The model under review builds one solid part; all positions refer to its coordinate system, in mm. Coordinates: 2 decimals unless noted, no trailing zeros. Write each loop counter-clockwise with the first axis right and the second up, starting at its lowest first coordinate (ties: lowest second). Pieces come first, ordered by that corner, then holes. Notation, with made-up numbers: (4, 22.25) - (23, 22.25) arc R19 ccw to (23, 31.25) - close; hole circle Ø5 at (58, -18.75). An arc over 180 degrees is marked (long way). Return JSON: item names as keys, results as strings. Group by question number.
(1) We need section A-A on z = 3.35. State the section outline as (x, y) points.
(2) We need section C-C on x = 47. State the section outline as (y, z) points.
(3) To check wall thickness, follow L1, parallel to Y at x = 65, z = 4.55; L2, parallel to Y at x = 109.5, z = 2.85; L3, parallel to X at y = -108, z = 3.4. State the ranges of each line that lie inside material, in increasing order. Write a range as from..to.
(4) We need section B-B on y = 101.5. State the section outline as (x, z) points.
(5) Draft analysis for pull direction Y (two halves, no side actions). For faces 1 (the face through (116, 13, 5)), 2 (the face through (50.7, 122.99, 2.54)), 3 (the face through (98.92, 14.67, 2.46)), state which applies: released by +Y, released by -Y, zero draft, split by the parting line, or undercut.
(6) For pin 1 Ø2 at (x, z) = (57, 4) entering from -Y; pin 2 Ø1 at (y, z) = (113, 2) entering from -X; pin 3 Ø1.5 at (x, z) = (78.5, 2) entering from +Y, all flat-tipped, find the tip position at first contact; note any pin that passes through.
```python
from build123d import *

# Parameters (mm, degrees)
BOSS_EXTRU_2_DEPTH      = 5
ENL_V_MAT_EXTRU_1_DEPTH = 10
ESQUISSE3_W             = 70.825033907
ESQUISSE3_H             = 52.172348309
ENL_V_MAT_EXTRU_2_DEPTH = 10
ESQUISSE4_R             = 2
ESQUISSE4_R_2           = 1.87013138
ENL_V_MAT_EXTRU_3_DEPTH = 10
ENL_V_MAT_EXTRU_4_DEPTH = 10


with BuildPart() as part:
    # Esquisse1 → Boss.-Extru.2 (new body)
    with BuildSketch(Plane.XY):
        with BuildLine():
            Line((-2, 166.988023523), (-2, 99.979998))
            ThreePointArc((-2, 99.979998), (100, 0), (-2, -99.979998))
            Line((-2, -99.979998), (-2, -166.988023523))
            ThreePointArc((-2, -166.988023523), (167, 0), (-2, 166.988023523))
        make_face()
    extrude(amount=BOSS_EXTRU_2_DEPTH)

    # Esquisse2 → Enlèv. mat.-Extru.1 (cut)
    with BuildSketch(Plane.XY.offset(5)):
        Polygon((29.390638032, 43.425593165), (38.112910781, 92.452182407), (63.648561005, 154.395144619), (68.028776979, 172.275239399), (-24.955464007, 192.914301625), (-14.988060504, 82.801476905), align=None)
        Polygon((56.192163409, 19.645406226), (29.390638032, 43.425593165), (-11.148286352, -184.437631398), (102.415881909, -156.025065414), (102.415881909, -133.007210905), (53.907034164, -84.226074749), align=None)
    extrude(amount=-ENL_V_MAT_EXTRU_1_DEPTH, mode=Mode.SUBTRACT)

    # Esquisse3 → Enlèv. mat.-Extru.2 (cut)
    with BuildSketch(Plane.XY.offset(5)):
        with Locations((-10.008332903, -121.270932698)):
            Rectangle(ESQUISSE3_W, ESQUISSE3_H)
    extrude(amount=-ENL_V_MAT_EXTRU_2_DEPTH, mode=Mode.SUBTRACT)

    # Esquisse4 → Enlèv. mat.-Extru.3 (cut)
    with BuildSketch(Plane.XY.offset(5)):
        with Locations((109.034633389, 14.54127648)):
            Circle(ESQUISSE4_R)
        with Locations((101.697400647, -41.92420186)):
            Circle(ESQUISSE4_R)
        with Locations((87.156124167, 67.11043153)):
            Circle(ESQUISSE4_R_2)
        with Locations((122.810902236, 94.564698974)):
            Circle(ESQUISSE4_R)
        with Locations((143.30088273, -59.075011711)):
            Circle(ESQUISSE4_R)
        with Locations((153.639710685, 20.489980494)):
            Circle(ESQUISSE4_R)
    extrude(amount=-ENL_V_MAT_EXTRU_3_DEPTH, mode=Mode.SUBTRACT)

    # Esquisse5 → Enlèv. mat.-Extru.4 (cut)
    with BuildSketch(Plane.XY.offset(5)):
        Polygon((61.009483209, -79.232840152), (101.798321541, -132.386184065), (46.643469874, -98.897205978), (43.215654561, -74.196784885), (51.84018638, -72.999910462), align=None)
    extrude(amount=-ENL_V_MAT_EXTRU_4_DEPTH, mode=Mode.SUBTRACT)


solid = part.part
```
Ans:
{
 "1": {"outline": "(38.11, 92.45) arc R100 cw to (61.01, -79.23) - (101.8, -132.39) arc R167 ccw to (63.65, 154.4) - close; hole circle Ø3.74 at (87.16, 67.11); hole circle Ø4 at (101.7, -41.92); hole circle Ø4 at (109.03, 14.54); hole circle Ø4 at (122.81, 94.56); hole circle Ø4 at (143.3, -59.08); hole circle Ø4 at (153.64, 20.49)"},
 "2": {"outline": "(88.27, 0) - (114.01, 0) - (114.01, 5) - (88.27, 5) - close"},
 "3": {"L1": "-84.43..-75.99, 75.99..153.83", "L2": "-126.09..12.6, 16.49..126.09", "L3": "83.08..127.38"},
 "4": {"outline": "(41.84, 0) - (132.62, 0) - (132.62, 5) - (41.84, 5) - close"},
 "5": {"face 1": "zero draft", "face 2": "released by +Y", "face 3": "undercut"},
 "6": {"pin 1": "y = 81.46", "pin 2": "x = 46.38", "pin 3": "y = 147.8"}
}
